Geometry check sheet. Reference: drawing and pictorial views, mm from the part's lowest x, y, z. A direction names the side the tool comes from. Round coordinates to 2 decimals unless told otherwise and drop trailing zeros. Loops run counter-clockwise (first coordinate to the right, second up) from the corner with the lowest first, then second, coordinate; pieces in that order, holes last. Notation, with made-up numbers: (14.25, 30) - (54.25, 30) arc R20 cw to (54.25, 48) - close; hole circle Ø11 at (45, 89.25). An arc over 180 degrees is marked (long way). Answer as CSV lines item,"result". Start each with the question number.
1) Cross-section at D-D on z = 22.5. Record the boundary of the cut face in (x, y) (1 decimal), and give its area (3 significant figures).
2) Draft check along Y on the marked faces 1, 2, 3 and 4. Enter one of: released by +Y, released by -Y, zero draft, split by the parting line, or undercut.
3) Cross-section at C-C on x = 21. Record the boundary of the cut face in (y, z) (1 decimal), and give its area (3 significant figures).
4) Depth check by flat-ended pin: P1, Ø6, axis at x = 9, z = 10, coming from the -Y side; P2, Ø3, axis at y = 4.5, z = 22.5, coming from the -X side; P3, Ø3, axis at y = 18.59, z = 22.5, coming from the +X side; P4, Ø1, axis at x = 29, z = 26.5, coming from the +Y side (1 decimal). Enter the tip coordinate at first touch or a pass-through.
5) Cross-section at B-B on y = 25. Record the boundary of the cut face in (x, z), and give its area (3 significant figures).
6) Cross-section at A-A on z = 3. Record the boundary of the cut face in (x, y) (1 decimal).
7) Access from +Z, -Z, +X, -X, +Y, -Y to the whole of each face (thin tool, end or side, straight path). Record for the marked faces 5 and 6.
8) Thickness scan on line 1 along X through (y, z) = (11, 15.5); line 2 along X through (y, z) = (14.5, 16) (1 decimal); line 3 along Y through (x, z) = (11, 14) (1 decimal). Record the ranges inside material, lowest first.
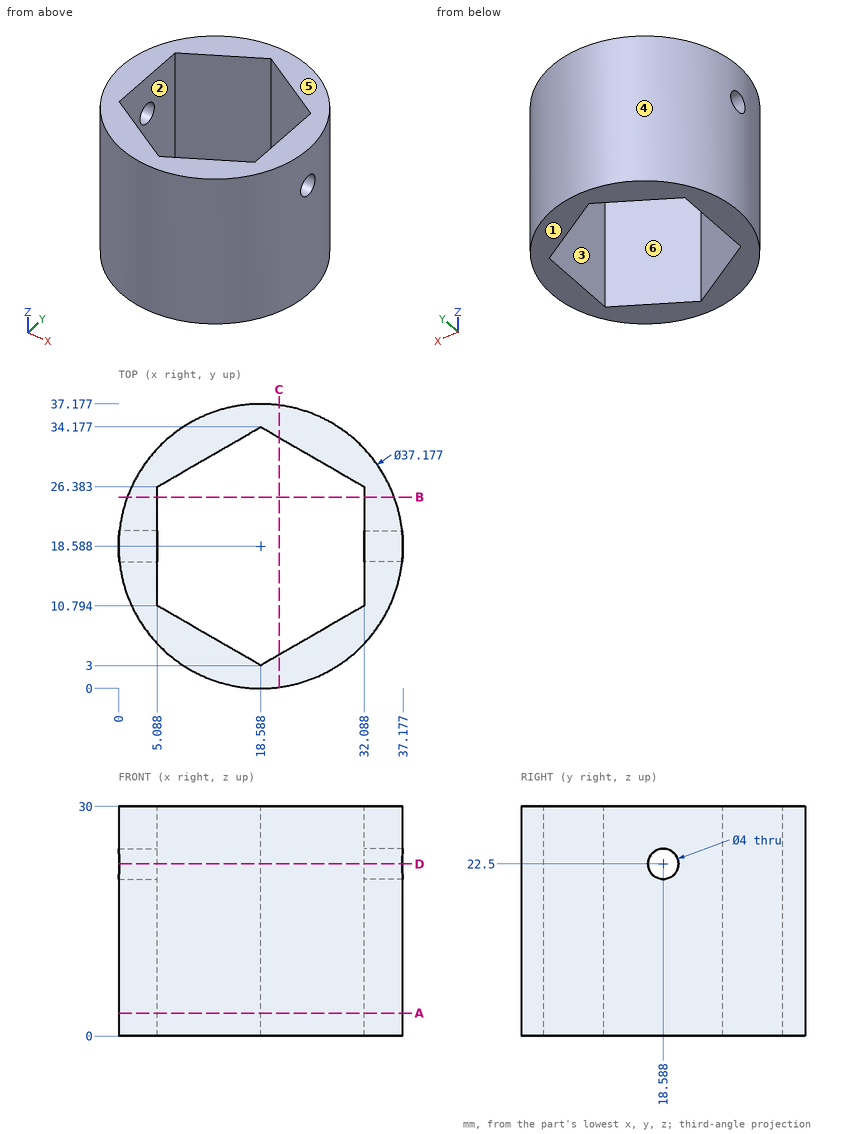
Answer block:
1,outline,"(0.1, 16.6) arc R18.6 ccw to (37.1, 16.6) - (32.1, 16.6) - (32.1, 10.8) - (18.6, 3) - (5.1, 10.8) - (5.1, 16.6) - close; (0.1, 20.6) - (5.1, 20.6) - (5.1, 26.4) - (18.6, 34.2) - (32.1, 26.4) - (32.1, 20.6) - (37.1, 20.6) arc R18.6 ccw to start"
1,area,"414 mm^2"
2,face 1,"zero draft"
2,face 2,"undercut"
2,face 3,"undercut"
2,face 4,"split by the parting line"
3,outline,"(0.2, 0) - (4.4, 0) - (4.4, 30) - (0.2, 30) - close; (32.8, 0) - (37, 0) - (37, 30) - (32.8, 30) - close"
3,area,"254 mm^2"
4,P1,"stops at y = 1.21"
4,P2,"stops at x = 4.91"
4,P3,"passes through"
4,P4,"stops at y = 34.3"
5,outline,"(1.14, 0) - (5.09, 0) - (5.09, 30) - (1.14, 30) - close; (32.09, 0) - (36.04, 0) - (36.04, 30) - (32.09, 30) - close"
5,area,"237 mm^2"
6,outline,"circle Ø37.2 at (18.6, 18.6); hole (5.1, 10.8) - (18.6, 3) - (32.1, 10.8) - (32.1, 26.4) - (18.6, 34.2) - (5.1, 26.4) - close"
7,face 5,"+Z, +X, -X, +Y, -Y"
7,face 6,"+Z, -Z"
8,line 1,"x = 1.62 to 5.09, 32.09 to 35.56"
8,line 2,"x = 0.5 to 5.1, 32.1 to 36.7"
8,line 3,"y = 1.6 to 7.4, 29.8 to 35.6"
